Design review of the part built by this model. Coordinates are the model's own, in mm. Face numbers are marked on the shaded views. A direction names the side the tool comes from. Round coordinates to 2 decimals unless told otherwise and drop trailing zeros. Order: outer loops, then holes, each group sorted by start corner. A loop starts at its lowest first (then second) coordinate and runs counter-clockwise, first axis right, second up. Notation, with made-up numbers: (37, 30.5) - (73, 30.5) arc R23 ccw to (73, 66.5) - close; hole circle Ø6 at (31.25, -16.5). An arc over 180 degrees is marked (long way). Use CSV: the item, a comma, the result in double quotes. Start each with the question number.
from build123d import *

# Parameters (mm, degrees)
F0_W      = 22.35
F0_H      = 16
F1_DEPTH  = 22.6
F2_W      = 19.35
F2_H      = 14.48
F3_DEPTH  = 2
F5_DEPTH  = 25
F6_W      = 3.5
F6_H      = 1.25
F7_DEPTH  = 2.18
F8_W      = 3.5
F8_H      = 1.25
F9_DEPTH  = 2.18
F10_W     = 3.5
F10_H     = 10.75
F11_DEPTH = 0.5
F12_W     = 14.5
F12_H     = 12.18
F13_DEPTH = 13.25
F14_W     = 11.5
F14_H     = 10.53
F15_DEPTH = 1.5
F16_W     = 3.58
F16_H     = 1
F17_DEPTH = 1.83
F18_W     = 3
F18_H     = 8.39
F19_DEPTH = 0.5
F20_W     = 3
F20_H     = 1.32
F21_DEPTH = 0.88
F22_W     = 3
F22_H     = 1.82
F23_DEPTH = 1.23
F24_R     = 2


with BuildPart() as f1:
    # F0 (on Front) → F1 (new body)
    with BuildSketch(Plane.XZ):
        with Locations((-2.416973, 8)):
            Rectangle(F0_W, F0_H)
    extrude(amount=F1_DEPTH)

    # F2 (on face) → F3 (cut)
    with BuildSketch(Plane.XZ.offset(22.6)):
        with Locations((-2.416973, 7.24)):
            Rectangle(F2_W, F2_H)
    extrude(amount=-F3_DEPTH, mode=Mode.SUBTRACT)

    # F4 (on face) → F5 (cut)
    with BuildSketch(Plane(origin=(-13.591973, 0, 0), x_dir=(0, -1, 0), z_dir=(-1, 0, 0))):
        Polygon((0, 16), (0, 14), (22.6, 16), align=None)
    extrude(amount=-F5_DEPTH, mode=Mode.SUBTRACT)

    # F6 (on face) → F7 (join)
    with BuildSketch(Plane(origin=(-13.591973, 0, 0), x_dir=(0, -1, 0), z_dir=(-1, 0, 0))):
        with Locations((20.85, 0.625)):
            Rectangle(F6_W, F6_H)
    extrude(amount=F7_DEPTH)

    # F8 (on face) → F9 (join)
    with BuildSketch(Plane.YZ.offset(8.758027)):
        with Locations((-20.85, 0.625)):
            Rectangle(F8_W, F8_H)
    extrude(amount=F9_DEPTH)

    # F10 (on face) → F11 (join)
    with BuildSketch(Plane(origin=(-13.591973, 0, 0), x_dir=(0, -1, 0), z_dir=(-1, 0, 0))):
        with Locations((20.85, 5.375)):
            Rectangle(F10_W, F10_H)
    extrude(amount=F11_DEPTH)

    # F12 (on face) → F13 (join)
    with BuildSketch(Plane(origin=(0, 0, 0), x_dir=(-1, 0, 0), z_dir=(0, 1, 0))):
        with Locations((2.416973, 6.09)):
            Rectangle(F12_W, F12_H)
    extrude(amount=F13_DEPTH)

    # F14 (on face) → F15 (cut)
    with BuildSketch(Plane(origin=(0, 13.25, 0), x_dir=(-1, 0, 0), z_dir=(0, 1, 0))):
        with Locations((2.416973, 5.265)):
            Rectangle(F14_W, F14_H)
    extrude(amount=-F15_DEPTH, mode=Mode.SUBTRACT)

    # F16 (on face) → F17 (join)
    with BuildSketch(Plane.XY.offset(12.18)):
        with Locations((-2.416973, 12.75)):
            Rectangle(F16_W, F16_H)
    extrude(amount=F17_DEPTH)

    # F18 (on face) → F19 (join)
    with BuildSketch(Plane.YZ.offset(4.833027)):
        with Locations((11.75, 4.195)):
            Rectangle(F18_W, F18_H)
    extrude(amount=F19_DEPTH)

    # F20 (on face) → F21 (join)
    with BuildSketch(Plane.YZ.offset(5.333027)):
        with Locations((11.75, 1.96)):
            Rectangle(F20_W, F20_H)
    extrude(amount=F21_DEPTH)

    # F22 (on face) → F23 (join)
    with BuildSketch(Plane(origin=(-9.666973, 0, 0), x_dir=(0, -1, 0), z_dir=(-1, 0, 0))):
        with Locations((-11.75, 2.21)):
            Rectangle(F22_W, F22_H)
    extrude(amount=F23_DEPTH)

    # F24
    f24_edges = [f1.edges().sort_by_distance(p)[0] for p in [
        (-13.591973, -11.3, 15),
        (8.758027, -11.3, 15),
        (4.833027, 6.625, 12.18),
        (-9.666973, 6.625, 12.18),
    ]]
    fillet(f24_edges, radius=F24_R)


solid = f1.part
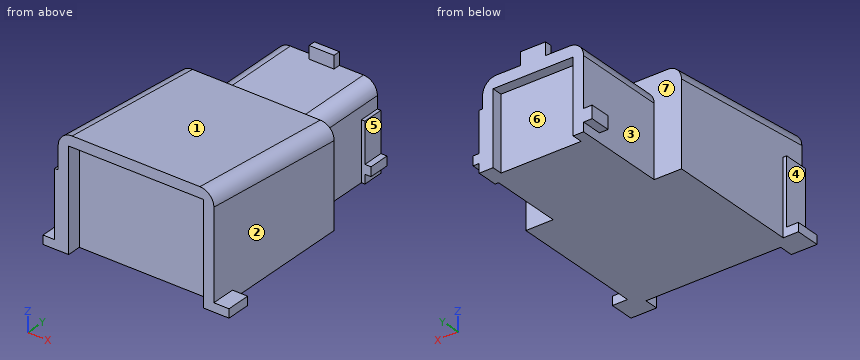
Q1. Take a section at A-A (z = 7.5). State the section outline as (x, y) points.
Q2. Take a section at B-B (x = 1). State the section outline as (y, z) points, plus the area to 3 significant figures.
Q3. Clearance check with flat-ended pins moving along their axes: pin 1 (1.5 mm diameter, centred on y = -7, z = 12, fed in from -X); pin 2 (1.5 mm diameter, centred on y = 11, z = 1.5, fed in from +X); pin 3 (0.5 mm diameter, centred on x = -3, y = 13, fed in from +Z); pin 4 (1.5 mm diameter, centred on x = 6.5, y = 6.5, fed in from +Z). State where each tip first meets the part, or that it passes through.
Q4. Take a section at D-D (x = -2). State the section outline as (y, z) points, plus the area to 3 significant figures.
Q5. For L1, parallel to X at y = -21, z = 9.75; L2, parallel to Y at x = -11.5, z = 9; L3, parallel to X at y = 4, z = 1, list the stretches that pass through material, from the lowest coordinate up. Write a range as [from, to].
Q6. Take a section at C-C (y = 1). State the section outline as (x, z) points.
Q7. Tool access review of the marked faces 4, 5, 6 and 7: name each direction out of +Z, -Z, +X, -X, +Y, -Y from which nothing blocks a thin tool from reaching the whole face with its end or side.
Q8. The part is to be moulded in two halves that separate along Y. For the marked faces 1, 2 and 3, say which applies: +Y half, -Y half, draft (parallel to the pull), parting line (faces both ways), or undercut.
Findings below:
1,outline,"(-14.09, -22.6) - (-12.09, -22.6) - (-12.09, -20.6) - (7.26, -20.6) - (7.26, -22.6) - (8.76, -22.6) - (8.76, 0) - (4.83, 0) - (4.83, 10.25) - (5.33, 10.25) - (5.33, 13.25) - (3.33, 13.25) - (3.33, 11.75) - (-8.17, 11.75) - (-8.17, 13.25) - (-9.67, 13.25) - (-9.67, 0) - (-13.59, 0) - (-13.59, -19.1) - (-14.09, -19.1) - close"
2,outline,"(-22.6, 14.48) - (-20.6, 14.48) - (-20.6, 0) - (11.75, 0) - (11.75, 10.53) - (13.25, 10.53) - (13.25, 12.18) - (0, 12.18) - (0, 14) - (-22.6, 16) - close"
2,area,"456 mm^2"
3,pin 1,"stops at x = -13.59"
3,pin 2,"stops at x = 6.21"
3,pin 3,"stops at z = 14.01"
3,pin 4,"passes through"
4,outline,"(-22.6, 14.48) - (-20.6, 14.48) - (-20.6, 0) - (11.75, 0) - (11.75, 10.53) - (13.25, 10.53) - (13.25, 14.01) - (12.25, 14.01) - (12.25, 12.18) - (0, 12.18) - (0, 14) - (-22.6, 16) - close"
4,area,"457 mm^2"
5,L1,"x = [-14.09, -12.09], [7.26, 8.76]"
5,L2,"y = [-20.6, 0]"
5,L3,"x = [-9.67, 4.83]"
6,outline,"(-9.67, 0) - (4.83, 0) - (4.83, 10.18) arc R2 ccw to (2.83, 12.18) - (-7.67, 12.18) arc R2 ccw to (-9.67, 10.18) - close"
7,face 4,"+Z, -X, +Y, -Y"
7,face 5,"+Z, +X, +Y"
7,face 6,"-Z, +Y"
7,face 7,"+Z"
8,face 1,"+Y half"
8,face 2,"draft"
8,face 3,"undercut"
